Here's how the part is built. I have some questions about the finished solid (model axes, mm). A direction names the side the tool comes from. Coordinates: 2 decimals unless noted, no trailing zeros. Loops run counter-clockwise (first coordinate to the right, second up) from the corner with the lowest first, then second, coordinate; pieces in that order, holes last. Notation, with made-up numbers: M 43.25,75.25 L 48.25,75.25 A23 ccw 48.25,93.25 Z; hole C 5.5,73.5 d7. An arc over 180 degrees is marked long. Use one line per item in the form item = value. Start each with the question number.
(1) Please list where these lines run through material, in increasing order: L1, parallel to X at y = 7.8, z = -36.5; L2, parallel to Z at x = 0, y = 6.45; L3, parallel to Y at x = 7, z = 32.
(2) On a 3-axis mill with a long thin cutter (end or side, diameter ignored), from which of +Z, -Z, +X, -X, +Y, -Y can I reach the whole of each face in a straight line? I mean faces 1 (the cylindrical face through (4.336, 2.465, 19.524)), 2 (the cylindrical face through (22, 7, 42)), 3 (the flat face through (0, 7, -47)). Say none if no direction works.
(3) Imagine slicing it at A-A, the plane x = 22. Please give me the cut outline in (y, z), and give its area (3 significant figures).
(4) Imagine slicing it at B-B, the plane z = -36.5. Please give me the cut outline in (x, y), and give its area (3 significant figures).
(5) Will this pin go through, and if not, where does the flat tip stop? P1, Ø1, axis at x = 25.5, z = 22.5, coming from the -Y side.
(6) Imagine slicing it at D-D, the plane z = 0. Please give me the cut outline in (x, y), and give its area (3 significant figures).
(7) Imagine slicing it at C-C, the plane y = 6. Please give me the cut outline in (x, z), and give its area (3 significant figures).
Autodesk Inventor part; units mm, degrees
ref_plane "YZ Plane" through (0, 0, 0) normal (1, 0, 0) x (0, 1, 0)
ref_plane "XZ Plane" through (0, 0, 0) normal (0, 1, 0) x (-1, 0, 0)
ref_plane "XY Plane" through (0, 0, 0) normal (0, 0, 1) x (1, 0, 0)
sketch "Sketch1" plane through (0, 0, 0) normal (0, 1, 0) x (-1, 0, 0)
  circle A0 centre (0, 0) radius 20
  dimension "d0" = 40
extrude "Extrusion1" add sketch "Sketch1" along normal blind 5
sketch "Sketch2" plane through (0, 5, 0) normal (0, 1, 0) x (1, 0, 0)
  line L0 (-32, -47) -> (32, -47)
  line L1 (32, -47) -> (32, 47)
  line L2 (32, 47) -> (-32, 47)
  line L3 (-32, 47) -> (-32, -47)
  line L4 (-32, -47) -> (32, 47) construction
  line L5 (32, -47) -> (-32, 47) construction
  line L6 (-22, -36.5) -> (22, -36.5) construction
  line L7 (22, -36.5) -> (22, 36.5) construction
  line L8 (22, 36.5) -> (-22, 36.5) construction
  line L9 (-22, 36.5) -> (-22, -36.5) construction
  line L10 (-22, -36.5) -> (22, 36.5) construction
  line L11 (22, -36.5) -> (-22, 36.5) construction
  line L12 (-22, 35.5) -> (-22, 37.5) construction
  line L13 (-17.5, 35.5) -> (-17.5, 37.5)
  line L14 (-26.5, 37.5) -> (-26.5, 35.5)
  arc A0 (-26.5, 35.5) -> (-17.5, 35.5) centre (-22, 35.5) ccw
  arc A1 (-17.5, 37.5) -> (-26.5, 37.5) centre (-22, 37.5) ccw
  line L15 (-32, 0) -> (32, 0) construction
  line L16 (0, 47) -> (0, -47) construction
  line L17 (17.5, 35.5) -> (17.5, 37.5)
  line L18 (26.5, 37.5) -> (26.5, 35.5)
  arc A2 (17.5, 35.5) -> (26.5, 35.5) centre (22, 35.5) ccw
  arc A3 (26.5, 37.5) -> (17.5, 37.5) centre (22, 37.5) ccw
  line L19 (-17.5, -35.5) -> (-17.5, -37.5)
  line L20 (-26.5, -37.5) -> (-26.5, -35.5)
  arc A4 (-17.5, -35.5) -> (-26.5, -35.5) centre (-22, -35.5) ccw
  arc A5 (-26.5, -37.5) -> (-17.5, -37.5) centre (-22, -37.5) ccw
  arc A6 (17.5, -37.5) -> (26.5, -37.5) centre (22, -37.5) ccw
  line L21 (26.5, -37.5) -> (26.5, -35.5)
  arc A7 (26.5, -35.5) -> (17.5, -35.5) centre (22, -35.5) ccw
  line L22 (17.5, -35.5) -> (17.5, -37.5)
  circle A8 centre (0, 36.5) radius 4.5
  circle A9 centre (0, -36.5) radius 4.5
  point P0 (0, 0)
  dimension "d3" = 64
  dimension "d4" = 94
  dimension "d5" = 44
  dimension "d6" = 73
  dimension "d7" = 1
  dimension "d8" = 9
  dimension "d9" = 9
  dimension "d10" = 9
extrude "Extrusion2" add sketch "Sketch2" along normal blind 4
properties part number "motor_bracket_upper" material "Steel, Alloy"
Answer:
q1.L1 = -32 to -26.5, -17.5 to -4.5, 4.5 to 17.5, 26.5 to 32
q1.L2 = -47 to -41, -32 to 32, 41 to 47
q1.L3 = 5 to 9
q2.face_1 = -Y
q2.face_2 = +Y, -Y
q2.face_3 = -Z, +X, -X, +Y, -Y
q3.outline = M 5,-47 L 9,-47 L 9,-42 L 5,-42 Z; M 5,-31 L 9,-31 L 9,31 L 5,31 Z; M 5,42 L 9,42 L 9,47 L 5,47 Z
q3.area = 288 mm²
q4.outline = M -32,5 L -26.5,5 L -26.5,9 L -32,9 Z; M -17.5,5 L -4.5,5 L -4.5,9 L -17.5,9 Z; M 4.5,5 L 17.5,5 L 17.5,9 L 4.5,9 Z; M 26.5,5 L 32,5 L 32,9 L 26.5,9 Z
q4.area = 148 mm²
q5.P1 = 5
q6.outline = M -32,5 L -20,5 L -20,0 L 20,0 L 20,5 L 32,5 L 32,9 L -32,9 Z
q6.area = 456 mm²
q7.outline = M -32,-47 L 32,-47 L 32,47 L -32,47 Z; hole M -26.5,-37.5 A4.5 ccw -17.5,-37.5 L -17.5,-35.5 A4.5 ccw -26.5,-35.5 Z; hole M -26.5,35.5 A4.5 ccw -17.5,35.5 L -17.5,37.5 A4.5 ccw -26.5,37.5 Z; hole C 0,-36.5 d9; hole C 0,36.5 d9; hole M 17.5,-37.5 A4.5 ccw 26.5,-37.5 L 26.5,-35.5 A4.5 ccw 17.5,-35.5 Z; hole M 17.5,35.5 A4.5 ccw 26.5,35.5 L 26.5,37.5 A4.5 ccw 17.5,37.5 Z
q7.area = 5,560 mm²
